Geometry check sheet. Reference: the model listing, model coordinates, mm. A direction names the side the tool comes from. Round coordinates to 2 decimals unless told otherwise and drop trailing zeros. Write each loop counter-clockwise with the first axis right and the second up, starting at its lowest first coordinate (ties: lowest second). Pieces come first, ordered by that corner, then holes. Notation, with made-up numbers: (29, 44) -> (79, 44) arc R27 cw to (79, 77) -> close; hole circle Ø6 at (77.25, 51.5). An arc over 180 degrees is marked (long way). Return JSON: item names as keys, results as strings. Group by question number.
Autodesk Inventor part; units mm, degrees
ref_plane "YZ Plane" through (0, 0, 0) normal (1, 0, 0) x (0, 1, 0)
ref_plane "XZ Plane" through (0, 0, 0) normal (0, 1, 0) x (-1, 0, 0)
ref_plane "XY Plane" through (0, 0, 0) normal (0, 0, 1) x (1, 0, 0)
sketch "Sketch1" plane through (0, 0, 0) normal (1, 0, 0) x (0, 1, 0)
  line L0 (1.7321, 1) -> (30, 1)
  line L1 (30, 1) -> (30, -1)
  line L2 (30, -1) -> (1.7321, -1)
  line L3 (-1.7321, 1) -> (-30, 1)
  line L4 (-30, 1) -> (-30, -1)
  line L5 (-30, -1) -> (-1.7321, -1)
  arc A0 (1.7321, 1) -> (-1.7321, 1) centre (0, 0) ccw
  arc A1 (-1.7321, -1) -> (1.7321, -1) centre (0, 0) ccw
  dimension "d1" = 2
  dimension "d26" = 30
  dimension "d27" = 30
extrude "Extrusion1" add sketch "Sketch1" along normal blind 30
properties part number "Flat Hinge"
1) Tool access check on faces 1 (the face through (30, 0, 0)), 2 (the face through (15, 16, -1)), 3 (the face through (15, -16, 1)), 4 (the face through (15, 16, 1)), 5 (the face through (15, -16, -1)). Record the directions out of +Z, -Z, +X, -X, +Y, -Y that give a thin tool (end or side, any length) a straight path to the whole face; none if there is none.
2) Sectioned sample at A-A on x = 20.25. Enter the section's corners in (y, z), and give its area (3 significant figures).
3) Material ranges on probe 1 along Z at (x, y) = (26.5, 13.5); probe 2 along Y at (x, z) = (17, 1.4); probe 3 along Y at (x, z) = (17.75, 1.65), recorded low to high. Write a range as [from, to].
4) Sectioned sample at B-B on y = 6. Enter the section's corners in (x, z).
5) Go/stop test with flat-tipped pins: P1, Ø10, axis at x = 25.5, y = -23.5, coming from the -Z side; P2, Ø1.5, axis at x = 10, y = -17.5, coming from the +Z side. Record where each tip stops, or that it passes through.
Evaluation:
{
 "1": {"face 1": "+Z, -Z, +X, +Y, -Y", "face 2": "-Z, +X, -X, +Y", "face 3": "+Z, +X, -X, -Y", "face 4": "+Z, +X, -X, +Y", "face 5": "-Z, +X, -X, -Y"},
 "2": {"outline": "(-30, -1) -> (-1.73, -1) arc R2 ccw to (1.73, -1) -> (30, -1) -> (30, 1) -> (1.73, 1) arc R2 ccw to (-1.73, 1) -> (-30, 1) -> close", "area": "125 mm2"},
 "3": {"probe 1": "z = [-1, 1]", "probe 2": "y = [-1.43, 1.43]", "probe 3": "y = [-1.13, 1.13]"},
 "4": {"outline": "(0, -1) -> (30, -1) -> (30, 1) -> (0, 1) -> close"},
 "5": {"P1": "stops at z = -1", "P2": "stops at z = 1"}
}
